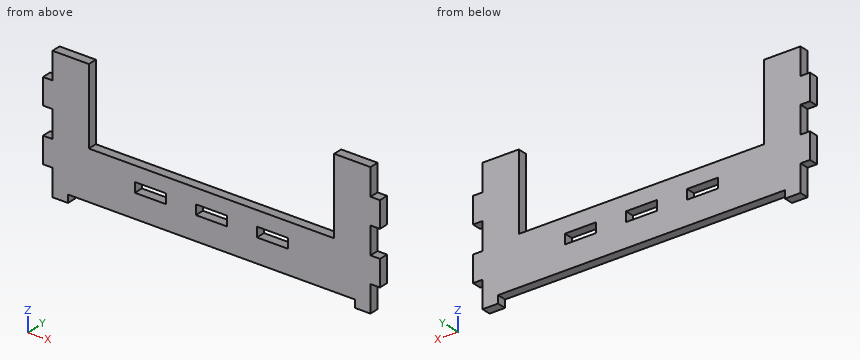
from build123d import *

# Parameters (mm, degrees)
BOSS_EXTRUDE1_DEPTH = 3
SKETCH2_W           = 3.2
SKETCH2_H           = 8.875
SKETCH2_W_2         = 10.2
SKETCH2_H_2         = 3.2
CUT_EXTRUDE1_DEPTH  = 4


with BuildPart() as part:
    # Sketch1 → Boss-Extrude1 (new body)
    with BuildSketch(Plane(origin=(0, 0, 0), x_dir=(1, 0, 0), z_dir=(0, 1, 0))):
        Polygon((-40.172217102, 0), (-55.172217102, 0), (-55.172217102, 43.95), (55.172217102, 43.95), (55.172217102, 0), (40.172217102, 0), (40.172217102, 25), (-40.172217102, 25), align=None)
    extrude(amount=-BOSS_EXTRUDE1_DEPTH)

    # Sketch2 → Cut-Extrude1 (cut, through all)
    with BuildSketch(Plane(origin=(0, 0, 0), x_dir=(1, 0, 0), z_dir=(0, 1, 0))):
        Polygon((-46.972217102, 40.85), (46.972217102, 40.85), (46.972217102, 43.35), (52.072217102, 43.35), (52.072217102, 34.6), (55.272217102, 34.6), (55.272217102, 44.05), (-55.272217102, 44.05), (-55.272217102, 34.6), (-52.072217102, 34.6), (-52.072217102, 43.35), (-46.972217102, 43.35), align=None)
        with Locations((-53.672217102, 21.6875)):
            Rectangle(SKETCH2_W, SKETCH2_H)
        with Locations((-53.672217102, 4.3375)):
            Rectangle(SKETCH2_W, SKETCH2_H)
        with Locations((53.672217102, 4.3375)):
            Rectangle(SKETCH2_W, SKETCH2_H)
        with Locations((53.672217102, 21.6875)):
            Rectangle(SKETCH2_W, SKETCH2_H)
        with Locations((-20, 31.5)):
            Rectangle(SKETCH2_W_2, SKETCH2_H_2)
        with Locations((20, 31.5)):
            Rectangle(SKETCH2_W_2, SKETCH2_H_2)
        with Locations((0, 31.5)):
            Rectangle(SKETCH2_W_2, SKETCH2_H_2)
    extrude(amount=-CUT_EXTRUDE1_DEPTH, mode=Mode.SUBTRACT)


solid = part.part
For this review, take the finished solid that the model builds, in its own axes (mm). Coordinates: 2 decimals unless noted, no trailing zeros. Loops run counter-clockwise (first coordinate to the right, second up) from the corner with the lowest first, then second, coordinate; pieces in that order, holes last. Notation, with made-up numbers: (-36, 89) - (-16, 89) arc R26 ccw to (-16, 108) - close; hole circle Ø3 at (20.5, 32). An arc over 180 degrees is marked (long way). Return JSON: item names as keys, results as strings.
Item 1: Take a section at B-B (x = -21). Give the boundary of the cut face in (y, z), then the cut area to 4 significant figures.
Determined:
{"outline": "(-3, -40.85) - (0, -40.85) - (0, -33.1) - (-3, -33.1) - close; (-3, -29.9) - (0, -29.9) - (0, -25) - (-3, -25) - close", "area": "37.95 mm2"}
Item 2: For line 1 (X direction, y = -1.1, z = -31); line 2 (Z direction, x = 2.5, y = -2.4); line 3 (X direction, y = -1.85, z = -3.5), list the stretches that pass through material, from the lowest coordinate up.
Determined:
{"line 1": "x = -55.17 to -25.1, -14.9 to -5.1, 5.1 to 14.9, 25.1 to 55.17", "line 2": "z = -40.85 to -33.1, -29.9 to -25", "line 3": "x = -52.07 to -40.17, 40.17 to 52.07"}
Item 3: Insertion check: pin 1 (1.5 mm diameter, centred on y = -0.5, z = -5.5, fed in from +X); pin 2 (1.5 mm diameter, centred on y = -1.5, z = -22.5, fed in from -X). Each pin has a flat end and moves straight along its axis. Give the tip position at first contact, or say it passes through.
Determined:
{"pin 1": "stops at x = 52.07", "pin 2": "stops at x = -52.07"}
Item 4: Take a section at A-A (z = -23). Give the boundary of the cut face in (x, y), then the cut area to 3 significant figures.
Determined:
{"outline": "(-52.07, -3) - (-40.17, -3) - (-40.17, 0) - (-52.07, 0) - close; (40.17, -3) - (52.07, -3) - (52.07, 0) - (40.17, 0) - close", "area": "71.4 mm2"}
Item 5: Take a section at C-C (z = -37.5). Give the boundary of the cut face in (x, y).
Determined:
{"outline": "(-52.07, -3) - (52.07, -3) - (52.07, 0) - (-52.07, 0) - close"}
Item 6: Take a section at D-D (y = -1.2). State how many separate pieces and enclosed holes the cut face has, then the cut area to 3 significant figures.
Determined:
{"separate pieces": "1", "enclosed holes": "3", "area": "2,280 mm2"}
